Answer from the drawing. Dimensions are ordinates in mm from the lowest x, y and z of the part. Coordinates: 2 decimals unless noted, no trailing zeros. Order: outer loops, then holes, each group sorted by start corner. A loop starts at its lowest first (then second) coordinate and runs counter-clockwise, first axis right, second up. Notation, with made-up numbers: (-19, 40) -> (34, 40) arc R29 ccw to (34, 79) -> close; hole circle Ø4 at (14.25, 44.25). An arc over 180 degrees is marked (long way). Answer in a Markdown table with one row per item.
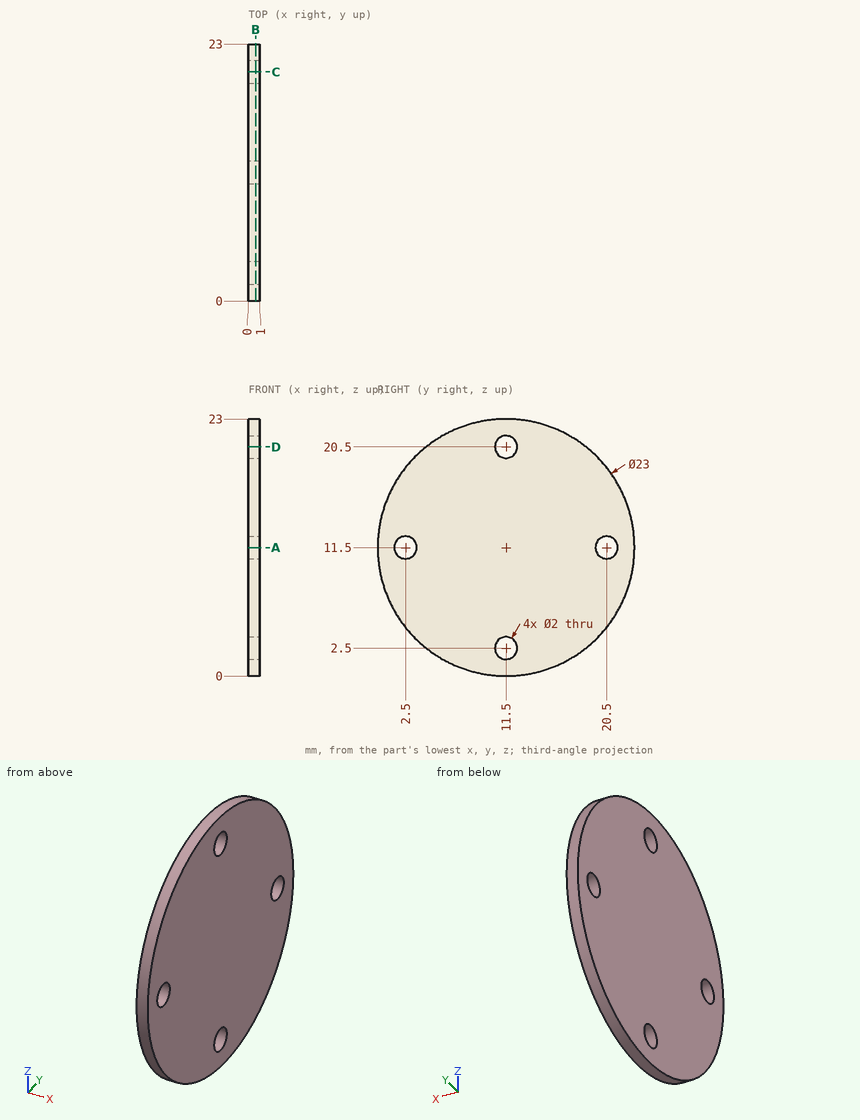
Q1. The part is cut by section B-B (x = 0.65). Write down the section's boundary in (y, z).
Outcome:
| item | result |
|---|---|
| outline | circle Ø23 at (11.5, 11.5); hole circle Ø2 at (2.5, 11.5); hole circle Ø2 at (11.5, 2.5); hole circle Ø2 at (11.5, 20.5); hole circle Ø2 at (20.5, 11.5) |
Q2. Consider line 1 (Z direction, x = 0.3, y = 2.5); line 2 (Z direction, x = 0.45, y = 17.5); line 3 (Y direction, x = 0.9, z = 5.25). Determine where each line is inside the solid, lowest interval first.
Outcome:
| item | result |
|---|---|
| line 1 | 4.34 to 10.5, 12.5 to 18.66 |
| line 2 | 1.69 to 21.31 |
| line 3 | 1.85 to 21.15 |
Q3. The part is cut by section A-A (z = 11.5). Write down the section's boundary in (x, y).
Outcome:
| item | result |
|---|---|
| outline | (0, 0) -> (1, 0) -> (1, 1.5) -> (0, 1.5) -> close; (0, 3.5) -> (1, 3.5) -> (1, 19.5) -> (0, 19.5) -> close; (0, 21.5) -> (1, 21.5) -> (1, 23) -> (0, 23) -> close |
Q4. The part is cut by section C-C (y = 20.5). Write down the section's boundary in (x, z).
Outcome:
| item | result |
|---|---|
| outline | (0, 4.34) -> (1, 4.34) -> (1, 10.5) -> (0, 10.5) -> close; (0, 12.5) -> (1, 12.5) -> (1, 18.66) -> (0, 18.66) -> close |
